Work out the finished part from the listing and answer in its coordinate system (mm). A direction names the side the tool comes from. Give positions to 0.01 mm unless a question says otherwise; leave off trailing zeros. Loops run counter-clockwise (first coordinate to the right, second up) from the corner with the lowest first, then second, coordinate; pieces in that order, holes last.
```python
from build123d import *

# Parameters (mm, degrees)
F1_DEPTH = 76.2
F2_R     = 25.7565229103
F3_DEPTH = 25.4


with BuildPart() as f1:
    # F0 (on Front) → F1 (new body)
    with BuildSketch(Plane.XZ):
        with BuildLine():
            Line((-217.0628905296, 44.0026623952), (-217.0628905296, 53.0386045575))
            Line((-217.0628905296, 53.0386045575), (-208.0269483673, 53.0386045575))
            ThreePointArc((-208.0269483673, 53.0386045575), (-223.452266507, 59.4279805349), (-217.0628905296, 44.0026623952))
        make_face()
        with BuildLine():
            ThreePointArc((78.9043606112, 53.0386045575), (27.5418888777, 104.401076291), (-23.8205828557, 53.0386045575))
            Line((-23.8205828557, 53.0386045575), (27.5418888777, 53.0386045575))
            Line((27.5418888777, 53.0386045575), (27.5418888777, 1.676132824))
            ThreePointArc((27.5418888777, 1.676132824), (63.860640939, 16.7198524963), (78.9043606112, 53.0386045575))
        make_face()
        with BuildLine():
            Line((-217.0628905296, -103.4866347909), (-217.0628905296, -78.593862027))
            ThreePointArc((-217.0628905296, -78.593862027), (-234.6647389535, -121.0884832148), (-192.1701177657, -103.4866347909))
            Line((-192.1701177657, -103.4866347909), (-217.0628905296, -103.4866347909))
        make_face()
        with BuildLine():
            ThreePointArc((38.0325649024, -103.4866347909), (34.959917034, -96.0686066346), (27.5418888777, -92.9959587662))
            Line((27.5418888777, -92.9959587662), (27.5418888777, -103.4866347909))
            Line((27.5418888777, -103.4866347909), (17.0512128531, -103.4866347909))
            ThreePointArc((17.0512128531, -103.4866347909), (27.5418888777, -113.9773108156), (38.0325649024, -103.4866347909))
        make_face()
        with BuildLine():
            Line((-208.0269483673, 53.0386045575), (-217.0628905296, 53.0386045575))
            Line((-217.0628905296, 53.0386045575), (-217.0628905296, 44.0026623952))
            ThreePointArc((-217.0628905296, 44.0026623952), (-210.6735145522, 46.6492285801), (-208.0269483673, 53.0386045575))
        make_face()
        with BuildLine():
            Line((27.5418888777, 53.0386045575), (-23.8205828557, 53.0386045575))
            ThreePointArc((-23.8205828557, 53.0386045575), (-8.7768631835, 16.7198524963), (27.5418888777, 1.676132824))
            Line((27.5418888777, 1.676132824), (27.5418888777, 53.0386045575))
        make_face()
        with BuildLine():
            ThreePointArc((-192.1701177657, -103.4866347909), (-199.4610421057, -85.884786367), (-217.0628905296, -78.593862027))
            Line((-217.0628905296, -78.593862027), (-217.0628905296, -103.4866347909))
            Line((-217.0628905296, -103.4866347909), (-192.1701177657, -103.4866347909))
        make_face()
        with BuildLine():
            Line((27.5418888777, -103.4866347909), (27.5418888777, -92.9959587662))
            ThreePointArc((27.5418888777, -92.9959587662), (20.1238607215, -96.0686066346), (17.0512128531, -103.4866347909))
            Line((17.0512128531, -103.4866347909), (27.5418888777, -103.4866347909))
        make_face()
        with BuildLine():
            Line((-23.8205828557, 53.0386045575), (-208.0269483673, 53.0386045575))
            ThreePointArc((-208.0269483673, 53.0386045575), (-210.6735145522, 46.6492285801), (-217.0628905296, 44.0026623952))
            Line((-217.0628905296, 44.0026623952), (-217.0628905296, -78.593862027))
            ThreePointArc((-217.0628905296, -78.593862027), (-199.4610421057, -85.884786367), (-192.1701177657, -103.4866347909))
            Line((-192.1701177657, -103.4866347909), (17.0512128531, -103.4866347909))
            ThreePointArc((17.0512128531, -103.4866347909), (20.1238607215, -96.0686066346), (27.5418888777, -92.9959587662))
            Line((27.5418888777, -92.9959587662), (27.5418888777, 1.676132824))
            ThreePointArc((27.5418888777, 1.676132824), (-8.7768631835, 16.7198524963), (-23.8205828557, 53.0386045575))
        make_face()
    extrude(amount=-F1_DEPTH)

    # F2 (on face) → F3 (cut)
    with BuildSketch(Plane.XY.offset(53.0386045575)):
        with Locations((-109.0174764395, 42.8577400744)):
            Circle(F2_R)
    extrude(amount=-F3_DEPTH, mode=Mode.SUBTRACT)


solid = f1.part
```
Q1. Section C-C on z = -65.5 is taken. Give the vertices of the cut face in (x, y), plus the area to 3 significant figures.
Q2. Section D-D on x = -72.5 is taken. Give the vertices of the cut face in (y, z).
Q3. Which of the six approach directions +Z, -Z, +X, -X, +Y, -Y give full straight-line access (tool end or side, diameter ignored) to faces 5 (the face through (-217.063, 38, -16)), 6 (the face through (-84, 76.2, -10)), 7 (the face through (27.542, 38, -46)), 8 (the face through (-135, 38, 53.039)), 9 (the face through (65.04, 37.57, 88.14))?
Q4. Consider line 1 along Z through (x, y) = (-63, 23.5); line 2 along Z through (x, y) = (27, 24); line 3 along X through (y, z) = (31, -42). Determine where each line is inside the solid, lowest interval first.
Q5. Determine the mould class of faces 1 (the face through (-84, 0, -10)), 2 (the face through (-89, 38, -103.487)), 3 (the face through (-109, 43, 27.639)), 4 (the face through (-95.171, 64.576, 40.516)) for opening direction Y: +Y half, -Y half, draft (parallel to the pull), parting line (faces both ways), or undercut.
Q6. Section B-B on x = -222 is taken. Give the vertices of the cut face in (y, z), plus the area to 3 significant figures.
Q7. Section A-A on y = 8 is taken. Give the vertices of the cut face in (x, z), plus the area to 3 significant figures.
Q8. Given pin 1 (6 mm diameter, centred on x = -189, y = 25, fed in from -Z); pin 2 (3 mm diameter, centred on x = 40, y = 25.5, fed in from +Z); pin 3 (3 mm diameter, centred on y = 57.5, z = 70, fed in from -X), each flat-ended and moving along its own axis, determine where each tip first touches the part or whether it passes through.
Check result:
1. outline: (-217.06, 0) - (27.54, 0) - (27.54, 76.2) - (-217.06, 76.2) - close
1. area: 18,600 mm2
2. outline: (0, -103.49) - (76.2, -103.49) - (76.2, 53.04) - (0, 53.04) - close
3. face 5: -X, +Y, -Y
3. face 6: +Z, -Z, +X, -X, +Y
3. face 7: +X, +Y, -Y
3. face 8: +Z, +Y, -Y
3. face 9: +Y, -Y
4. line 1: z = -103.49 to 53.04
4. line 2: z = -113.96 to 104.4
4. line 3: x = -217.06 to 27.54
5. face 1: -Y half
5. face 2: draft
5. face 3: undercut
5. face 4: undercut
6. outline: (0, -127.88) - (76.2, -127.88) - (76.2, -79.09) - (0, -79.09) - close; (0, 45.47) - (76.2, 45.47) - (76.2, 60.61) - (0, 60.61) - close
6. area: 4,870 mm2
7. outline: (-217.06, -78.59) arc R24.89 ccw (long way) to (-192.17, -103.49) - (17.05, -103.49) arc R10.49 ccw (long way) to (27.54, -93) - (27.54, 1.68) arc R51.36 ccw (long way) to (-23.82, 53.04) - (-208.03, 53.04) arc R9.04 ccw (long way) to (-217.06, 44) - close
7. area: 46,400 mm2
8. pin 1: stops at z = -103.49
8. pin 2: stops at z = 103.22
8. pin 3: stops at x = -21.44
